```python
from build123d import *

# Parameters (mm, degrees)
BOSS_EXTRUDE1_DEPTH        = 4.7625
SKETCH2_R                  = 11.90625
CUT_EXTRUDE1_DEPTH         = 97.524699721
M6_CLEARANCE_HOLE1_D       = 6.4
SKETCH5_R                  = 9.525
CUT_EXTRUDE2_DEPTH         = 97.524699721
FILLET1_R                  = 3.175
F_10_CLEARANCE_HOLE1_D     = 4.9784
F_10_CLEARANCE_HOLE1_DEPTH = 9.525
F_10_CLEARANCE_HOLE1_TIP   = 1.495662253


with BuildPart() as part:
    # Sketch1 → Boss-Extrude1 (new body)
    with BuildSketch(Plane(origin=(0, 0, 0), x_dir=(1, 0, 0), z_dir=(0, 1, 0))):
        with BuildLine():
            Line((4.7625, 28.175329967), (78.845833333, 15.652961093))
            ThreePointArc((78.845833333, 15.652961093), (92.075, 0), (78.845833333, -15.652961093))
            Line((78.845833333, -15.652961093), (4.7625, -28.175329967))
            ThreePointArc((4.7625, -28.175329967), (-15.889172282, -23.750049035), (-27.86051193, -6.35))
            Line((-27.86051193, -6.35), (-50.8, -6.35))
            Line((-50.8, -6.35), (-50.8, 6.35))
            Line((-50.8, 6.35), (-27.86051193, 6.35))
            ThreePointArc((-27.86051193, 6.35), (-15.889172282, 23.750049035), (4.7625, 28.175329967))
        make_face()
    extrude(amount=BOSS_EXTRUDE1_DEPTH)

    # Sketch2 → Cut-Extrude1 (cut, through all)
    with BuildSketch(Plane(origin=(0, 4.7625, 0), x_dir=(1, 0, 0), z_dir=(0, 1, 0))):
        with Locations(Location((76.2, 0, 0), (0, 0, 270))):
            Circle(SKETCH2_R)
    extrude(amount=-CUT_EXTRUDE1_DEPTH, mode=Mode.SUBTRACT)

    # M6 Clearance Hole1 (through all)
    with Locations(Plane(origin=(0, 4.7625, -17.5), x_dir=(0, 0, 1), z_dir=(0, 1, 0))):
        with Locations((0, 0), (26.25, -15.155444566), (26.25, 15.155444566)):
            Hole(M6_CLEARANCE_HOLE1_D / 2)

    # Sketch5 → Cut-Extrude2 (cut, through all)
    with BuildSketch(Plane(origin=(0, 4.7625, 0), x_dir=(1, 0, 0), z_dir=(0, 1, 0))):
        with Locations(Location((0, 0, 0), (0, 0, 270))):
            Circle(SKETCH5_R)
    extrude(amount=-CUT_EXTRUDE2_DEPTH, mode=Mode.SUBTRACT)

    # Fillet1
    fillet1_edges = [part.edges().sort_by_distance(p)[0] for p in [
        (-27.86051193, 2.38125, 6.35),
        (-27.86051193, 2.38125, -6.35),
    ]]
    fillet(fillet1_edges, radius=FILLET1_R)

    # #10 Clearance Hole1
    with Locations(Plane(origin=(-45.974, 4.7625, 0), x_dir=(0, 0, 1), z_dir=(0, 1, 0))):
        with Locations((0, 0)):
            Hole(F_10_CLEARANCE_HOLE1_D / 2, depth=F_10_CLEARANCE_HOLE1_DEPTH)
            with Locations((0, 0, -(F_10_CLEARANCE_HOLE1_DEPTH + F_10_CLEARANCE_HOLE1_TIP / 2))):  # 118° drill point
                Cone(0, F_10_CLEARANCE_HOLE1_D / 2, F_10_CLEARANCE_HOLE1_TIP, mode=Mode.SUBTRACT)


solid = part.part
```
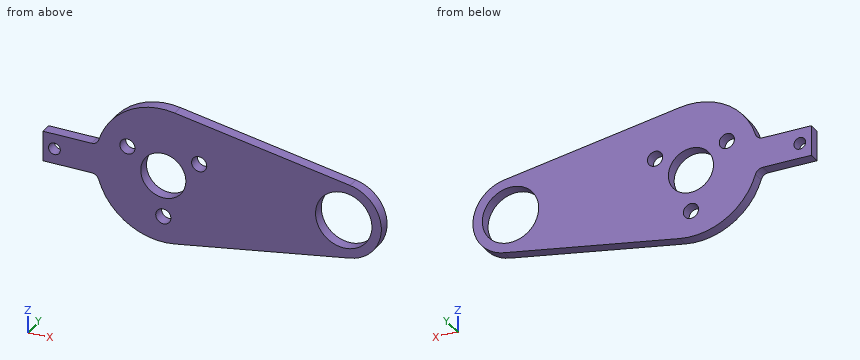
Read the model definition and answer for the solid it produces. Units are mm, in the model's axes. Give positions to 0.01 mm unless a question says otherwise; leave off trailing zeros. Order: outer loops, then holes, each group sorted by start corner. A loop starts at its lowest first (then second) coordinate and runs counter-clockwise, first axis right, second up. Notation, with made-up numbers: (-33.5, 71.5) -> (9.5, 71.5) arc R23 ccw to (9.5, 95.5) -> close; hole circle Ø8 at (70, -20.75). An arc over 180 degrees is marked (long way). One line per item, written item: value. Start each with the question number.
(1) The part is cut by section D-D (x = 70). Determine the outline of the cut face in (y, z), and give its area (3 significant figures).
(2) The part is cut by section B-B (z = -17.5). Determine the outline of the cut face in (x, y), and give its area (3 significant figures).
(3) The part is cut by section A-A (z = 0). Determine the outline of the cut face in (x, y) (1 decimal).
(4) The part is cut by section C-C (y = 0.95). State how many separate pieces and enclosed holes the cut face has, and give its area (3 significant figures).
(5) Flat-ended cylindrical pins translate along their axes: P1, Ø1.5, axis at x = 30, y = 4, coming from the +Z side; P2, Ø6, axis at x = 61, z = -22, coming from the -Y side; P3, Ø1, axis at y = 2.5, z = -11.5, coming from the +X side; P4, Ø1.4, axis at x = -36.5, y = 3.5, coming from the -Z side. Find the tip coordinate at first contact, or state that the pin passes through.
(6) Straight lines are drawn through the part: L1, parallel to X at y = 2.25, z = 8.75; L2, parallel to Z at x = 63, y = 4; L3, parallel to Z at x = 79.5, y = 2.9. For each, find the intervals that lie inside material, in ascending order.
Taken from the geometry:
1. outline: (0, -17.15) -> (4.76, -17.15) -> (4.76, -10.16) -> (0, -10.16) -> close; (0, 10.16) -> (4.76, 10.16) -> (4.76, 17.15) -> (0, 17.15) -> close
1. area: 66.5 mm^2
2. outline: (-22.59, 0) -> (-3.2, 0) -> (-3.2, 4.76) -> (-22.59, 4.76) -> close; (3.2, 0) -> (67.92, 0) -> (67.92, 4.76) -> (3.2, 4.76) -> close
2. area: 401 mm^2
3. outline: (-50.8, 0) -> (-48.5, 0) -> (-48.5, 4.8) -> (-50.8, 4.8) -> close; (-43.5, 0) -> (-9.5, 0) -> (-9.5, 4.8) -> (-43.5, 4.8) -> close; (9.5, 0) -> (64.3, 0) -> (64.3, 4.8) -> (9.5, 4.8) -> close; (88.1, 0) -> (92.1, 0) -> (92.1, 4.8) -> (88.1, 4.8) -> close
4. separate pieces: 1
4. enclosed holes: 6
4. area: 4,550 mm^2
5. P1: z = 24.04
5. P2: through
5. P3: x = 87.65
5. P4: z = -6.35
6. L1: -27.2 to -18.36, -11.96 to -3.76, 3.76 to 11.96, 18.36 to 68.13, 84.27 to 89.45
6. L2: -18.33 to 18.33
6. L3: -15.53 to -11.44, 11.44 to 15.53
